```python
from build123d import *

# Parameters (mm, degrees)
MAIN_EXTRUSION_DEPTH                                 = 24.5
FRONT_CAVE_DEPTH                                     = 10
SKETCH2_W                                            = 14
SKETCH2_H                                            = 14
SKETCH2_W_2                                          = 8.5
SKETCH2_H_2                                          = 18
KEY_CUTOUTS_DEPTH                                    = 3
CUT_EXTRUDE1_DEPTH                                   = 11.5
CSK_FOR_M2_5_COUNTERSUNK_FLAT_HEAD_SCREW_D           = 2.9
CSK_FOR_M2_5_COUNTERSUNK_FLAT_HEAD_SCREW_CSINK_D     = 5.5
CSK_FOR_M2_5_COUNTERSUNK_FLAT_HEAD_SCREW_CSINK_ANGLE = 90
CUT_EXTRUDE2_DEPTH                                   = 2
CUT_EXTRUDE3_DEPTH                                   = 2
FILLET1_R                                            = 1
SKETCH9_W                                            = 8
SKETCH9_H                                            = 21
CUT_EXTRUDE4_DEPTH                                   = 41
SKETCH10_W                                           = 6
SKETCH10_H                                           = 10
CUT_EXTRUDE5_DEPTH                                   = 10.75
CUT_EXTRUDE6_DEPTH                                   = 1.5
SKETCH13_W                                           = 3.2
SKETCH13_H                                           = 60
CUT_EXTRUDE8_DEPTH                                   = 7
SKETCH15_W                                           = 7
SKETCH15_H                                           = 21
CUT_EXTRUDE9_DEPTH                                   = 3


with BuildPart() as part:
    # Sketch1 → Main Extrusion (new body)
    with BuildSketch(Plane.XY):
        with BuildLine():
            Line((-61.875, -60), (61.875, -60))
            ThreePointArc((61.875, -60), (63.996320344, -59.121320344), (64.875, -57))
            Line((64.875, -57), (64.875, 57))
            ThreePointArc((64.875, 57), (63.996320344, 59.121320344), (61.875, 60))
            Line((61.875, 60), (-61.875, 60))
            ThreePointArc((-61.875, 60), (-63.996320344, 59.121320344), (-64.875, 57))
            Line((-64.875, 57), (-64.875, -57))
            ThreePointArc((-64.875, -57), (-63.996320344, -59.121320344), (-61.875, -60))
        make_face()
    extrude(amount=MAIN_EXTRUSION_DEPTH)

    # Sketch3 → Front Cave (cut)
    with BuildSketch(Plane.XY.offset(24.5)):
        with BuildLine():
            Line((-64.875, 48), (50.875, 48))
            ThreePointArc((50.875, 48), (52.289213562, 47.414213562), (52.875, 46))
            Line((52.875, 46), (52.875, -46))
            ThreePointArc((52.875, -46), (52.289213562, -47.414213562), (50.875, -48))
            Line((50.875, -48), (-64.875, -48))
            Line((-64.875, -48), (-64.875, 48))
        make_face()
    extrude(amount=-FRONT_CAVE_DEPTH, mode=Mode.SUBTRACT)

    # Sketch2 → Key Cutouts (cut)
    with BuildSketch(Plane.XY.offset(14.5)):
        with Locations((-52.375, -0.1)):
            Rectangle(SKETCH2_W, SKETCH2_H)
        with Locations((-52.375, 38)):
            Rectangle(SKETCH2_W, SKETCH2_H)
        with Locations((-33.325, 38)):
            Rectangle(SKETCH2_W, SKETCH2_H)
        with Locations((-14.275, 38)):
            Rectangle(SKETCH2_W, SKETCH2_H)
        with Locations((4.775, 38)):
            Rectangle(SKETCH2_W, SKETCH2_H)
        with Locations((23.825, 38)):
            Rectangle(SKETCH2_W, SKETCH2_H)
        with Locations((42.875, 38)):
            Rectangle(SKETCH2_W, SKETCH2_H)
        with Locations((18.584400006, -38.05)):
            Rectangle(SKETCH2_W_2, SKETCH2_H_2)
        with Locations((-52.375, 18.95)):
            Rectangle(SKETCH2_W, SKETCH2_H)
        with Locations((-33.325, 18.95)):
            Rectangle(SKETCH2_W, SKETCH2_H)
        with Locations((-14.275, 18.95)):
            Rectangle(SKETCH2_W, SKETCH2_H)
        with Locations((4.775, 18.95)):
            Rectangle(SKETCH2_W, SKETCH2_H)
        with Locations((23.825, 18.95)):
            Rectangle(SKETCH2_W, SKETCH2_H)
        with Locations((42.875, 18.95)):
            Rectangle(SKETCH2_W, SKETCH2_H)
        with Locations((-33.325, -0.1)):
            Rectangle(SKETCH2_W, SKETCH2_H)
        with Locations((-14.275, -0.1)):
            Rectangle(SKETCH2_W, SKETCH2_H)
        with Locations((4.775, -0.1)):
            Rectangle(SKETCH2_W, SKETCH2_H)
        with Locations((23.825, -0.1)):
            Rectangle(SKETCH2_W, SKETCH2_H)
        with Locations((42.875, -0.1)):
            Rectangle(SKETCH2_W, SKETCH2_H)
        with Locations((-52.375, -19.15)):
            Rectangle(SKETCH2_W, SKETCH2_H)
        with Locations((-33.325, -19.15)):
            Rectangle(SKETCH2_W, SKETCH2_H)
        with Locations((-14.275, -19.15)):
            Rectangle(SKETCH2_W, SKETCH2_H)
        with Locations((4.775, -19.15)):
            Rectangle(SKETCH2_W, SKETCH2_H)
        with Locations((23.825, -19.15)):
            Rectangle(SKETCH2_W, SKETCH2_H)
        with Locations((42.875, -19.15)):
            Rectangle(SKETCH2_W, SKETCH2_H)
        with Locations((-26.063, -38.2)):
            Rectangle(SKETCH2_W, SKETCH2_H)
        with Locations((-49.875, -38.2)):
            Rectangle(SKETCH2_W, SKETCH2_H)
        with Locations((-2.251, -38.2)):
            Rectangle(SKETCH2_W, SKETCH2_H)
        with Locations((31.084, -38.15)):
            Rectangle(SKETCH2_W, SKETCH2_H)
        with Locations((43.583599994, -38.05)):
            Rectangle(SKETCH2_W_2, SKETCH2_H_2)
    extrude(amount=-KEY_CUTOUTS_DEPTH, mode=Mode.SUBTRACT)

    # Sketch4 → Cut-Extrude1 (cut)
    with BuildSketch(Plane.XY):
        Polygon((-64.875, 55), (54.375, 55), (54.375, 17.5), (59.875, 17.5), (59.875, -55), (-64.875, -55), align=None)
    extrude(amount=CUT_EXTRUDE1_DEPTH, mode=Mode.SUBTRACT)

    # CSK for M2.5 Countersunk Flat Head Screw1 (through all)
    with Locations(Plane(origin=(-42.85, 28.475, 14.5), x_dir=(1, 0, 0), z_dir=(0, 0, 1))):
        with Locations((0, 0), (76.2, 0), (76.2, -38.1), (0, -38.1)):
            CounterSinkHole(CSK_FOR_M2_5_COUNTERSUNK_FLAT_HEAD_SCREW_D / 2, CSK_FOR_M2_5_COUNTERSUNK_FLAT_HEAD_SCREW_CSINK_D / 2, counter_sink_angle=CSK_FOR_M2_5_COUNTERSUNK_FLAT_HEAD_SCREW_CSINK_ANGLE)

    # Sketch6 → Cut-Extrude2 (cut)
    with BuildSketch(Plane.XZ.offset(60)):
        Polygon((-44.875, 0), (-36.875, 7), (64.875, 7), (64.875, 0), align=None)
    extrude(amount=-CUT_EXTRUDE2_DEPTH, mode=Mode.SUBTRACT)

    # Sketch8 → Cut-Extrude3 (cut)
    with BuildSketch(Plane(origin=(64.875, 0, 0), x_dir=(0, 0, -1), z_dir=(1, 0, 0))):
        Polygon((0, -60), (-7, -60), (-7, 32), (0, 40), align=None)
    extrude(amount=-CUT_EXTRUDE3_DEPTH, mode=Mode.SUBTRACT)

    # Fillet1
    fillet1_edges = [part.edges().sort_by_distance(p)[0] for p in [
        (63.996320344, 59.121320344, 24.5),
        (0, 60, 24.5),
        (-63.996320344, 59.121320344, 24.5),
        (-64.875, 52.5, 24.5),
        (-64.875, -52.5, 24.5),
        (-63.996320344, -59.121320344, 24.5),
        (0, -60, 24.5),
        (-7, -48, 24.5),
        (52.289213562, -47.414213562, 24.5),
        (52.875, 0, 24.5),
        (52.289213562, 47.414213562, 24.5),
        (-7, 48, 24.5),
        (63.996320344, -59.121320344, 24.5),
        (62.875, -58, 3.5),
        (64.875, 0, 24.5),
    ]]
    fillet(fillet1_edges, radius=FILLET1_R)

    # Sketch9 → Cut-Extrude4 (cut)
    with BuildSketch(Plane(origin=(0, 60, 0), x_dir=(1, 0, 0), z_dir=(0, 1, 0))):
        with Locations((57.875, -11.75)):
            Rectangle(SKETCH9_W, SKETCH9_H)
    extrude(amount=-CUT_EXTRUDE4_DEPTH, mode=Mode.SUBTRACT)

    # Sketch10 → Cut-Extrude5 (cut)
    with BuildSketch(Plane(origin=(0, 0, 11.5), x_dir=(-1, 0, 0), z_dir=(0, 0, -1))):
        with Locations((-56.875, 12.5)):
            Rectangle(SKETCH10_W, SKETCH10_H)
    extrude(amount=-CUT_EXTRUDE5_DEPTH, mode=Mode.SUBTRACT)

    # Sketch11 → Cut-Extrude6 (cut)
    with BuildSketch(Plane(origin=(0, 19, 0), x_dir=(1, 0, 0), z_dir=(0, 1, 0))):
        with BuildLine():
            Line((59.875, -6.25), (59.875, -17.25))
            ThreePointArc((59.875, -17.25), (57.875, -19.25), (55.875, -17.25))
            Line((55.875, -17.25), (55.875, -6.25))
            ThreePointArc((55.875, -6.25), (57.875, -4.25), (59.875, -6.25))
        make_face()
    extrude(amount=-CUT_EXTRUDE6_DEPTH, mode=Mode.SUBTRACT)

    # Sketch13 → Cut-Extrude8 (cut)
    with BuildSketch(Plane(origin=(0, 0, 11.5), x_dir=(-1, 0, 0), z_dir=(0, 0, -1))):
        with Locations((-58.275, -25)):
            Rectangle(SKETCH13_W, SKETCH13_H)
    extrude(amount=-CUT_EXTRUDE8_DEPTH, mode=Mode.SUBTRACT)

    # Sketch15 → Cut-Extrude9 (cut)
    with BuildSketch(Plane(origin=(0, 60, 0), x_dir=(1, 0, 0), z_dir=(0, 1, 0))):
        with Locations((50.375, -11.75)):
            Rectangle(SKETCH15_W, SKETCH15_H)
    extrude(amount=-CUT_EXTRUDE9_DEPTH, mode=Mode.SUBTRACT)


solid = part.part
```
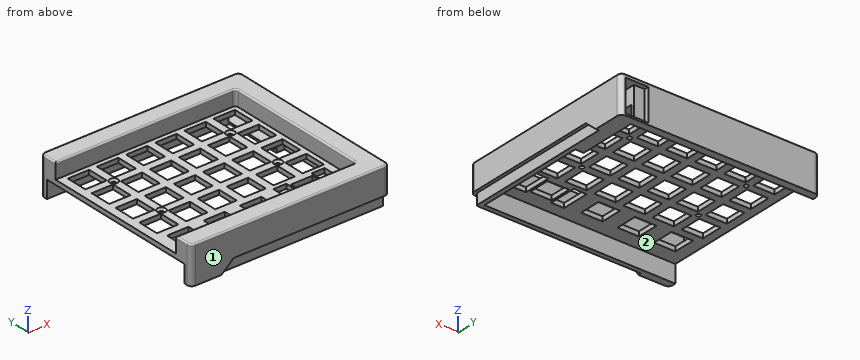
Check sheet for the modelled part. Datum: model origin and axes. Units: mm. Face numbers are marked on the shaded views. A direction names the side the tool comes from. Give positions to 0.01 mm unless a question says otherwise; leave off trailing zeros. Loops run counter-clockwise (first coordinate to the right, second up) from the corner with the lowest first, then second, coordinate; pieces in that order, holes last. Notation, with made-up numbers: (84.5, 72.25) - (95.5, 72.25) arc R31 cw to (95.5, 105.25) - close; hole circle Ø5 at (51.5, 26.25). An arc over 180 degrees is marked (long way). One line per question, with ' | ' between items. Start each with the question number.
1. Gauge pin test, flat ends, axial feed: pin 1 Ø5 at (x, y) = (55.5, 13) entering from -Z; pin 2 Ø7.5 at (x, y) = (53.5, 45.5) entering from +Z; pin 3 Ø8 at (x, y) = (-5.5, 1) entering from +Z; pin 4 Ø12 at (y, z) = (25, 5) entering from -X (3 decimals). Record the tip position at first contact, or that the pin passes through.
2. Cross-section at A-A, the plane x = -14.5. Give the number of separate pieces and of enclosed holes in the cut face, plus the area to 3 significant figures.
3. Cross-section at C-C, the plane y = -51. Enter the section's corners in (x, z) (3 decimals), plus the area to 3 significant figures.
4. Set-up check for the marked faces 1 and 2: record each of +Z, -Z, +X, -X, +Y, -Y from which the full face is reachable in a straight line by a thin tool's end or side.
5. Material ranges on line 1 along Y through (x, z) = (33.35, 12.7) (3 decimals); line 2 along Y through (x, z) = (-31.5, 13); line 3 along Y through (x, z) = (-54, 1.5), recorded low to high. Write a range as [from, to].
Check result:
1) pin 1: stops at z = 11.5 | pin 2: stops at z = 24.5 | pin 3: stops at z = 14.5 | pin 4: stops at x = 54.375
2) separate pieces: 5 | enclosed holes: 0 | area: 532 mm2
3) outline: (-64.875, 11.5) - (56.675, 11.5) - (56.675, 18.5) - (59.875, 18.5) - (59.875, 0) - (62.875, 0) - (62.875, 7) - (64.875, 7) - (64.875, 23.5) arc R1 ccw to (63.875, 24.5) - (-63.875, 24.5) arc R1 ccw to (-64.875, 23.5) - close | area: 1,710 mm2
4) face 1: +Z, -Z, +X, -X, -Y | face 2: -Z, -X
5) line 1: y = [-60, -45.15], [-31.15, -11.075], [-8.175, 27.025], [29.925, 60] | line 2: y = [-60, -45.2], [-31.2, -26.15], [-12.15, -7.1], [6.9, 11.95], [25.95, 31], [45, 60] | line 3: y = [-60, -55], [55, 60]
